```python
from build123d import *

# Parameters (mm, degrees)
SKETCH_R        = 1.45
PAD001_DEPTH    = 1.6
SKETCH001_R     = 1.45
PAD002_DEPTH    = 13.75
POCKET_DEPTH    = 15
SKETCH003_R     = 1.45
PAD003_DEPTH    = 3.4
POCKET001_DEPTH = 5
POCKET002_DEPTH = 10


with BuildPart() as part:
    # Sketch → Pad001 (new body)
    with BuildSketch(Plane.XY):
        with BuildLine():
            Line((12.25, 182), (190.25, 182))
            ThreePointArc((196.25, 176), (194.492641, 180.242641), (190.25, 182))
            Line((196.25, 176), (196.25, 3))
            ThreePointArc((190.25, -3), (194.492641, -1.242641), (196.25, 3))
            Line((190.25, -3), (12.25, -3))
            ThreePointArc((6.25, 3), (8.007359, -1.242641), (12.25, -3))
            Line((6.25, 3), (6.25, 97))
            Line((23.25, 97), (6.25, 97))
            ThreePointArc((23.25, 97), (28.906854, 99.343146), (31.25, 105))
            Line((31.25, 122), (31.25, 105))
            ThreePointArc((31.25, 122), (28.906854, 127.656854), (23.25, 130))
            Line((6.25, 130), (23.25, 130))
            Line((6.25, 130), (6.25, 176))
            ThreePointArc((12.25, 182), (8.007359, 180.242641), (6.25, 176))
        make_face()
        with Locations((11, 173.49762)):
            Circle(SKETCH_R, mode=Mode.SUBTRACT)
        with Locations((11, 89.49762)):
            Circle(SKETCH_R, mode=Mode.SUBTRACT)
        with Locations((180.742493, 173.605331)):
            Circle(SKETCH_R, mode=Mode.SUBTRACT)
        with Locations((181.761108, 91.056091)):
            Circle(SKETCH_R, mode=Mode.SUBTRACT)
        with Locations((24.67, 76.67)):
            Circle(SKETCH_R, mode=Mode.SUBTRACT)
        with Locations((24.67, 24.67)):
            Circle(SKETCH_R, mode=Mode.SUBTRACT)
        with Locations((191.67, 24.67)):
            Circle(SKETCH_R, mode=Mode.SUBTRACT)
        with Locations((191.67, 76.67)):
            Circle(SKETCH_R, mode=Mode.SUBTRACT)
        with BuildLine():
            ThreePointArc((40.25, 97.49762), (42.593146, 91.840766), (48.25, 89.49762))
            Line((168.624548, 89.49762), (48.25, 89.49762))
            ThreePointArc((168.624548, 89.49762), (174.281402, 91.840766), (176.624548, 97.49762))
            Line((176.624548, 122), (176.624548, 97.49762))
            ThreePointArc((176.624548, 122), (174.281402, 127.656854), (168.624548, 130))
            Line((48.25, 130), (168.624548, 130))
            ThreePointArc((48.25, 130), (42.593146, 127.656854), (40.25, 122))
            Line((40.25, 97.49762), (40.25, 122))
        make_face(mode=Mode.SUBTRACT)
        with BuildLine():
            ThreePointArc((15.25, 147), (17.593146, 141.343146), (23.25, 139))
            Line((168.563514, 139), (23.25, 139))
            ThreePointArc((168.563514, 139), (174.220369, 141.343146), (176.563514, 147))
            Line((176.563514, 165.49762), (176.563514, 147))
            ThreePointArc((176.563514, 165.49762), (174.220369, 171.154474), (168.563514, 173.49762))
            Line((23.25, 173.49762), (168.563514, 173.49762))
            ThreePointArc((23.25, 173.49762), (17.593146, 171.154474), (15.25, 165.49762))
            Line((15.25, 147), (15.25, 165.49762))
        make_face(mode=Mode.SUBTRACT)
        with BuildLine():
            ThreePointArc((28.92, 14), (31.263146, 8.343146), (36.92, 6))
            Line((179.42, 6), (36.92, 6))
            ThreePointArc((179.42, 6), (185.076854, 8.343146), (187.42, 14))
            Line((187.42, 68.67), (187.42, 14))
            ThreePointArc((187.42, 68.67), (185.076854, 74.326854), (179.42, 76.67))
            Line((36.92, 76.67), (179.42, 76.67))
            ThreePointArc((36.92, 76.67), (31.263146, 74.326854), (28.92, 68.67))
            Line((28.92, 14), (28.92, 68.67))
        make_face(mode=Mode.SUBTRACT)
    extrude(amount=-PAD001_DEPTH)

    # Sketch001 → Pad002 (join)
    with BuildSketch(Plane.XY):
        with BuildLine():
            ThreePointArc((28.92, 76.67), (24.67, 80.92), (20.42, 76.67))
            Line((20.42, 76.67), (20.42, 6))
            ThreePointArc((20.42, 6), (24.67, 1.75), (28.92, 6))
            Line((28.92, 6), (28.92, 76.67))
        make_face()
        with Locations((24.67, 24.67)):
            Circle(SKETCH001_R, mode=Mode.SUBTRACT)
        with Locations((24.67, 76.67)):
            Circle(SKETCH001_R, mode=Mode.SUBTRACT)
        with BuildLine():
            ThreePointArc((196.25, 76.67), (191.835, 81.085), (187.42, 76.67))
            Line((187.42, 76.67), (187.42, 6))
            ThreePointArc((187.42, 6), (191.835, 1.585), (196.25, 6))
            Line((196.25, 6), (196.25, 76.67))
        make_face()
        with Locations((191.67, 76.67)):
            Circle(SKETCH001_R, mode=Mode.SUBTRACT)
        with Locations((191.67, 24.67)):
            Circle(SKETCH001_R, mode=Mode.SUBTRACT)
    extrude(amount=PAD002_DEPTH)

    # Sketch002 (on Face56 of Pad002) → Pocket (cut)
    with BuildSketch(Plane.YZ.offset(196.25)):
        with BuildLine():
            ThreePointArc((31, 22), (28.87868, 21.12132), (28, 19))
            Line((28, 9), (28, 19))
            ThreePointArc((28, 9), (28.87868, 6.87868), (31, 6))
            Line((61, 6), (31, 6))
            ThreePointArc((61, 6), (63.12132, 6.87868), (64, 9))
            Line((64, 19), (64, 9))
            ThreePointArc((64, 19), (63.12132, 21.12132), (61, 22))
            Line((31, 22), (61, 22))
        make_face()
    extrude(amount=-POCKET_DEPTH, mode=Mode.SUBTRACT)

    # Sketch003 → Pad003 (join)
    with BuildSketch(Plane.XY.offset(-0.1)):
        with BuildLine():
            ThreePointArc((185.508165, 93.637), (179.180199, 94.803148), (178.014051, 88.475182))
            Line((178.014051, 88.475182), (187.922943, 74.089091))
            ThreePointArc((187.922943, 74.089091), (194.250909, 72.922943), (195.417057, 79.250909))
            Line((195.417057, 79.250909), (185.508165, 93.637))
        make_face()
        with Locations((191.67, 76.67)):
            Circle(SKETCH003_R, mode=Mode.SUBTRACT)
        with Locations((181.761108, 91.056091)):
            Circle(SKETCH003_R, mode=Mode.SUBTRACT)
        with BuildLine():
            ThreePointArc((13.908197, 92.596796), (7.900824, 92.405817), (8.091803, 86.398444))
            Line((8.091803, 86.398444), (21.761803, 73.570824))
            ThreePointArc((21.761803, 73.570824), (27.769176, 73.761803), (27.578197, 79.769176))
            Line((27.578197, 79.769176), (13.908197, 92.596796))
        make_face()
        with Locations((24.67, 76.67)):
            Circle(SKETCH003_R, mode=Mode.SUBTRACT)
        with Locations((11, 89.49762)):
            Circle(SKETCH003_R, mode=Mode.SUBTRACT)
        with BuildLine():
            ThreePointArc((15.25, 173.49762), (11, 177.74762), (6.75, 173.49762))
            Line((6.75, 173.49762), (6.75, 165.49762))
            ThreePointArc((6.75, 165.49762), (11, 161.24762), (15.25, 165.49762))
            Line((15.25, 165.49762), (15.25, 173.49762))
        make_face()
        with Locations((11, 173.49762)):
            Circle(SKETCH003_R, mode=Mode.SUBTRACT)
        with BuildLine():
            ThreePointArc((180.742493, 178.155224), (176.1926, 173.605331), (180.742493, 169.055438))
            Line((180.742493, 169.055438), (191.700107, 169.055438))
            ThreePointArc((191.700107, 169.055438), (196.25, 173.605331), (191.700107, 178.155224))
            Line((191.700107, 178.155224), (180.742493, 178.155224))
        make_face()
        with Locations((180.742493, 173.605331)):
            Circle(SKETCH003_R, mode=Mode.SUBTRACT)
    extrude(amount=PAD003_DEPTH)

    # Sketch004 → Pocket001 (cut)
    with BuildSketch(Plane.XY):
        with BuildLine():
            ThreePointArc((75.723694, 140.85524), (75.016587, 140.562347), (74.723694, 139.85524))
            Line((74.723694, 134.85524), (74.723694, 139.85524))
            ThreePointArc((74.723694, 134.85524), (75.016587, 134.148133), (75.723694, 133.85524))
            Line((91.423694, 133.85524), (75.723694, 133.85524))
            ThreePointArc((91.423694, 133.85524), (92.130801, 134.148133), (92.423694, 134.85524))
            Line((92.423694, 139.85524), (92.423694, 134.85524))
            ThreePointArc((92.423694, 139.85524), (92.130801, 140.562347), (91.423694, 140.85524))
            Line((75.723694, 140.85524), (91.423694, 140.85524))
        make_face()
        with BuildLine():
            ThreePointArc((129.923694, 140.85524), (129.216587, 140.562347), (128.923694, 139.85524))
            Line((128.923694, 134.85524), (128.923694, 139.85524))
            ThreePointArc((128.923694, 134.85524), (129.216587, 134.148133), (129.923694, 133.85524))
            Line((145.623694, 133.85524), (129.923694, 133.85524))
            ThreePointArc((145.623694, 133.85524), (146.330801, 134.148133), (146.623694, 134.85524))
            Line((146.623694, 139.85524), (146.623694, 134.85524))
            ThreePointArc((146.623694, 139.85524), (146.330801, 140.562347), (145.623694, 140.85524))
            Line((129.923694, 140.85524), (145.623694, 140.85524))
        make_face()
    extrude(amount=-POCKET001_DEPTH, mode=Mode.SUBTRACT)

    # Sketch008 → Pocket002 (cut, symmetric)
    with BuildSketch(Plane.XY):
        with BuildLine():
            ThreePointArc((20.42, 3), (22.177359, -1.242641), (26.42, -3))
            Line((26.42, -33), (26.42, -3))
            Line((-9.58, -33), (26.42, -33))
            Line((-9.58, 84), (-9.58, -33))
            Line((20.42, 84), (-9.58, 84))
            Line((20.42, 3), (20.42, 84))
        make_face()
    extrude(amount=POCKET002_DEPTH, both=True, mode=Mode.SUBTRACT)


with BuildPart() as part_1:
    # Body001 placement: moved
    add(part.part.moved(Location((0, 0, -3.4))))


solid = part_1.part
```
Part model, mm, in its own coordinate system. A direction names the side the tool comes from. Round coordinates to 2 decimals unless told otherwise and drop trailing zeros. Loops run counter-clockwise (first coordinate to the right, second up) from the corner with the lowest first, then second, coordinate; pieces in that order, holes last. Notation, with made-up numbers: (-14, -25.75) -> (3, -25.75) arc R29 cw to (3, 12.25) -> close; hole circle Ø6 at (85.25, 2.5). An arc over 180 degrees is marked (long way). Use one line per item in the form item = value. Start each with the question number.
Item 1: Band-saw the part on A-A (y = 43). List the corners of the cut face in (x, z).
Item 2: Two-plate mould, pull along Y, no slides. Class faces 1 (the flat face through (182.651, 81.743, -1.773)), 2 (the flat face through (11, 170, -0.1)), 3 (the flat face through (102.6, 138.7, -3.4)): released by +Y, released by -Y, zero draft, split by the parting line, or undercut.
Item 3: Tool access for faces 4 (the cylindrical face through (28.844, 99.281, -4.189)), 5 (the cylindrical face through (10.91, 161.25, -1.77)), 6 (the flat face through (190.532, 86.343, -1.773)), 7 (the cylindrical face through (31.201, 8.406, -4.189)), 8 (the cylindrical face through (24.58, 1.75, 3.38)): list every direction of +Z, -Z, +X, -X, +Y, -Y with a clear straight run to the whole face (end or side of a thin tool).
Item 4: Drill centre lines: line 1 along X through (y, z) = (25, 0.5); line 2 along X through (y, z) = (12, 4); line 3 along X through (y, z) = (76.67, -1.7). Where is each one in solid material? Low to high.
Item 5: Drop flat-ended pins along their axis: pin 1 Ø5.5 at (x, y) = (187.5, 87) entering from +Z; pin 2 Ø3.5 at (x, y) = (11, 89.5) entering from -Z; pin 3 Ø1.1 at (y, z) = (31.5, 8.5) entering from -X; pin 4 Ø2.5 at (x, y) = (190.5, 50.5) entering from +Z. Give the stop position or say it passes through.
Item 6: Band-saw the part on B-B (x = 52). List the corners of the cut face in (y, z).
Data:
q1.outline = (20.42, -5) -> (28.92, -5) -> (28.92, 10.35) -> (20.42, 10.35) -> close; (187.42, -5) -> (196.25, -5) -> (196.25, 2.6) -> (187.42, 2.6) -> close
q2.face_1 = released by -Y
q2.face_2 = zero draft
q2.face_3 = undercut
q3.face_4 = +Z, -Z, -X
q3.face_5 = +Z
q3.face_6 = +Z, +X
q3.face_7 = +Z, -Z
q3.face_8 = +Z, -Y
q4.line_1 = 20.42 to 23.26, 26.08 to 28.92, 187.42 to 190.26, 193.08 to 196.25
q4.line_2 = 20.42 to 28.92, 187.42 to 196.25
q4.line_3 = 20.42 to 23.22, 26.12 to 28.92, 186.15 to 190.22, 193.12 to 196.25
q5.pin_1 = -0.1
q5.pin_2 = -5
q5.pin_3 = 20.42
q5.pin_4 = 2.6
q6.outline = (-3, -5) -> (6, -5) -> (6, -3.4) -> (-3, -3.4) -> close; (76.67, -5) -> (89.5, -5) -> (89.5, -3.4) -> (76.67, -3.4) -> close; (130, -5) -> (139, -5) -> (139, -3.4) -> (130, -3.4) -> close; (173.5, -5) -> (182, -5) -> (182, -3.4) -> (173.5, -3.4) -> close
